Source: CAD feature listing. Evaluate the final solid. Frame: model axes, mm. Face numbers are marked on the shaded views. A direction names the side the tool comes from. Round coordinates to 2 decimals unless told otherwise and drop trailing zeros. Answer as a JSON object with one key per item and string values.
from build123d import *

# Parameters (mm, degrees)
ESTRUSIONE_ESTRUSIONE1_DEPTH   = 7.5
ESTRUSIONE_ESTRUSIONE1_2_DEPTH = 7.5
SCHIZZO2_W                     = 31.4
SCHIZZO2_H                     = 19.45
ESTRUSIONE_ESTRUSIONE2_DEPTH   = 2
TAGLIO_ESTRUSIONE3_DEPTH       = 2.4
SCHIZZO5_3_R                   = 1.75
TAGLIO_ESTRUSIONE4_DEPTH       = 27.523810222
RACCORDO1_R                    = 1


with BuildPart() as part:
    # Schizzo1 → Estrusione-Estrusione1 (new body)
    with BuildSketch(Plane.XY):
        with BuildLine():
            Line((31.4, 19.45), (31.4, 6.5))
            Line((31.4, 6.5), (17.4, 6.5))
            Line((17.4, 6.5), (15, 6.5))
            Line((15, 6.5), (15, 13.5))
            Line((15, 13.5), (17.4, 13.5))
            ThreePointArc((17.4, 13.5), (17.694149412, 13.584360941), (17.898876404, 13.811797753))
            ThreePointArc((17.898876404, 13.811797753), (17.957611714, 13.961937846), (17.991456891, 14.119565217))
            ThreePointArc((17.991456891, 14.119565217), (18.041268354, 14.212771412), (18.140175425, 14.25))
            Line((18.140175425, 14.25), (18.4, 14.25))
            Line((18.4, 14.25), (18.659824575, 14.25))
            ThreePointArc((18.659824575, 14.25), (18.758731646, 14.212771412), (18.808543109, 14.119565217))
            ThreePointArc((18.808543109, 14.119565217), (18.842388286, 13.961937846), (18.901123596, 13.811797753))
            ThreePointArc((18.901123596, 13.811797753), (19.4, 13.5), (19.898876404, 13.811797753))
            ThreePointArc((19.898876404, 13.811797753), (19.957611714, 13.961937846), (19.991456891, 14.119565217))
            ThreePointArc((19.991456891, 14.119565217), (20.041268354, 14.212771412), (20.140175425, 14.25))
            Line((20.140175425, 14.25), (20.4, 14.25))
            Line((20.4, 14.25), (20.659824575, 14.25))
            ThreePointArc((20.659824575, 14.25), (20.758731646, 14.212771412), (20.808543109, 14.119565217))
            ThreePointArc((20.808543109, 14.119565217), (20.842388286, 13.961937846), (20.901123596, 13.811797753))
            ThreePointArc((20.901123596, 13.811797753), (21.4, 13.5), (21.898876404, 13.811797753))
            ThreePointArc((21.898876404, 13.811797753), (21.957611714, 13.961937846), (21.991456891, 14.119565217))
            ThreePointArc((21.991456891, 14.119565217), (22.041268354, 14.212771412), (22.140175425, 14.25))
            Line((22.140175425, 14.25), (22.4, 14.25))
            Line((22.4, 14.25), (22.659824575, 14.25))
            ThreePointArc((22.659824575, 14.25), (22.758731646, 14.212771412), (22.808543109, 14.119565217))
            ThreePointArc((22.808543109, 14.119565217), (22.842388286, 13.961937846), (22.901123596, 13.811797753))
            ThreePointArc((22.901123596, 13.811797753), (23.4, 13.5), (23.898876404, 13.811797753))
            ThreePointArc((23.898876404, 13.811797753), (23.957611714, 13.961937846), (23.991456891, 14.119565217))
            ThreePointArc((23.991456891, 14.119565217), (24.041268354, 14.212771412), (24.140175425, 14.25))
            Line((24.140175425, 14.25), (24.4, 14.25))
            Line((24.4, 14.25), (24.659824575, 14.25))
            ThreePointArc((24.659824575, 14.25), (24.758731646, 14.212771412), (24.808543109, 14.119565217))
            ThreePointArc((24.808543109, 14.119565217), (24.842388286, 13.961937846), (24.901123596, 13.811797753))
            ThreePointArc((24.901123596, 13.811797753), (25.4, 13.5), (25.898876404, 13.811797753))
            ThreePointArc((25.898876404, 13.811797753), (25.957611714, 13.961937846), (25.991456891, 14.119565217))
            ThreePointArc((25.991456891, 14.119565217), (26.041268354, 14.212771412), (26.140175425, 14.25))
            Line((26.140175425, 14.25), (26.4, 14.25))
            Line((26.4, 14.25), (26.659824575, 14.25))
            ThreePointArc((26.659824575, 14.25), (26.758731646, 14.212771412), (26.808543109, 14.119565217))
            ThreePointArc((26.808543109, 14.119565217), (26.842388286, 13.961937846), (26.901123596, 13.811797753))
            ThreePointArc((26.901123596, 13.811797753), (27.4, 13.5), (27.898876404, 13.811797753))
            ThreePointArc((27.898876404, 13.811797753), (27.957611714, 13.961937846), (27.991456891, 14.119565217))
            ThreePointArc((27.991456891, 14.119565217), (28.041268354, 14.212771412), (28.140175425, 14.25))
            Line((28.140175425, 14.25), (28.4, 14.25))
            Line((28.4, 14.25), (28.4, 14.95))
            Line((28.4, 14.95), (15, 14.95))
            add(Edge.make_bspline(
                [(15, 14.95), (14.198625643, 14.95), (12.206107526, 15.352992529), (5.436685448, 10.879393873), (0, 10.725)],
                knots=[0, 0, 0, 0, 0.57277107, 1, 1, 1, 1], degree=3))
            Line((0, 10.725), (0, 19.45))
            Line((0, 19.45), (31.4, 19.45))
        make_face()
    extrude(amount=ESTRUSIONE_ESTRUSIONE1_DEPTH)



with BuildPart() as body_2:
    # Schizzo1 → Estrusione-Estrusione1 2 (new body)
    with BuildSketch(Plane.XY):
        with BuildLine():
            Line((31.4, 4.5), (31.4, 0))
            Line((31.4, 0), (0, 0))
            Line((0, 0), (0, 8.725))
            add(Edge.make_bspline(
                [(15, 4.5), (14.198625643, 4.5), (12.206107526, 4.097007471), (5.436685448, 8.570606127), (0, 8.725)],
                knots=[0, 0, 0, 0, 0.57277107, 1, 1, 1, 1], degree=3))
            Line((15, 4.5), (31.4, 4.5))
        make_face()
    extrude(amount=ESTRUSIONE_ESTRUSIONE1_2_DEPTH)


with BuildPart() as part_1:
    add(part.part)

    add(body_2.part)  # Estrusione-Estrusione2 merges body 2
    # Schizzo2 → Estrusione-Estrusione2 (add)
    with BuildSketch(Plane(origin=(0, 0, 0), x_dir=(-1, 0, 0), z_dir=(0, 0, -1))):
        with Locations((-15.7, 9.725)):
            Rectangle(SCHIZZO2_W, SCHIZZO2_H)
    extrude(amount=ESTRUSIONE_ESTRUSIONE2_DEPTH)

    # Schizzo5 → Taglio-Estrusione3 (cut)
    with BuildSketch(Plane.ZY.offset(-15)):
        Polygon((5.308845727, 7.1), (6.983161507, 10), (5.366580754, 12.8), (5.308845727, 12.9), (5.308845727, 13.5), (2.191154273, 13.5), (2.191154273, 12.9), (0.516838493, 10), (1.980206835, 7.46537168), (1.980206835, 7.2), (1.980206835, 6.5), (5.308845727, 6.5), align=None)
    extrude(amount=-TAGLIO_ESTRUSIONE3_DEPTH, mode=Mode.SUBTRACT)

    # Schizzo5_3 → Taglio-Estrusione4 (cut, through all)
    with BuildSketch(Plane.ZY.offset(-15)):
        with Locations(Location((3.75, 10, 0), (0, 0, 270))):
            Circle(SCHIZZO5_3_R)
    extrude(amount=-TAGLIO_ESTRUSIONE4_DEPTH, mode=Mode.SUBTRACT)

    # Raccordo1
    raccordo1_edges = [part_1.edges().sort_by_distance(p)[0] for p in [
        (15, 13.5, 6.404422863),
        (15, 13.5, 1.095577137),
        (15, 6.5, 0.990103418),
        (15, 6.5, 6.404422863),
    ]]
    fillet(raccordo1_edges, radius=RACCORDO1_R)


solid = part_1.part
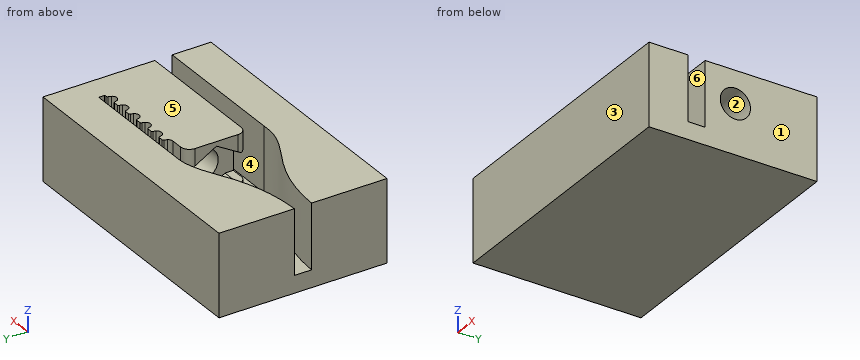
Item 1: Access query for the marked faces 1 and 2. Directions: +Z, -Z, +X, -X, +Y, -Y. A direction counts if a zero-diameter tool reaches every point of the face in a straight line with its end or side. Return the directions, or none.
Answer sheet:
{"face 1": "+Z, -Z, +X, +Y, -Y", "face 2": "+X"}
Item 2: Line query: probe 1 along Y at (x, z) = (16, 6.75); probe 2 along Z at (x, y) = (22.5, 10); probe 3 along Y at (x, z) = (19, 7). Output: solid intervals per line, ascending. Write a range as from..to.
Answer sheet:
{"probe 1": "y = 0..4.5, 6.5..9.6, 10.4..13.5, 14.95..19.45", "probe 2": "z = -2..2, 5.5..7.5", "probe 3": "y = 0..4.5, 6.5..13.67, 14.95..19.45"}
Item 3: Section A-A on z = 3.75. Give the number of separate pieces and of enclosed holes in the cut face, then the cut area to 3 significant figures.
Answer sheet:
{"separate pieces": "3", "enclosed holes": "0", "area": "409 mm²"}
Item 4: Pull-direction query (Y, two-part tool) for the marked faces 3, 4, 5 and 6; classes: pulls with the +Y half, pulls with the -Y half, needs draft (parallel to the pull), parting line crosses it, or undercut.
Answer sheet:
{"face 3": "pulls with the -Y half", "face 4": "undercut", "face 5": "needs draft", "face 6": "undercut"}
